Design review of the part built by this model. Coordinates are the model's own, in mm. A direction names the side the tool comes from. Give positions to 0.01 mm unless a question says otherwise; leave off trailing zeros. Loops run counter-clockwise (first coordinate to the right, second up) from the corner with the lowest first, then second, coordinate; pieces in that order, holes last. Notation, with made-up numbers: (58.25, 10.25) -> (82.25, 10.25) arc R9 cw to (82.25, 20.25) -> close; hole circle Ø9 at (13, -35.5). An arc over 180 degrees is marked (long way). Answer in a Markdown table with one row per item. Add a question column.
(1) For faces 1 (the flat face through (-15.24, 12, -2)), 2 (the flat face through (-16, -7, -3.175)), list the 3-axis set-ups (+Z, -Z, +X, -X, +Y, -Y) from which the entire face can be reached by the end or side of a thin tool; tool diameter is ignored.
(2) For line 1 (Y direction, x = -25.4, z = -0.95); line 2 (Y direction, x = 0, z = -2.4); line 3 (X direction, y = 6.5, z = -2) (3 decimals), list the stretches that pass through material, from the lowest coordinate up.
(3) Consider section D-D on y = 6.35. Write out the cut boundary in (x, z) (3 decimals), then the cut area to 3 significant figures.
(4) Consider section C-C on x = 12.7. Write out the cut boundary in (y, z) (3 decimals), then the cut area to 3 significant figures.
(5) Draft analysis for pull direction Y (two halves, no side actions). For faces 3 (the cylindrical face through (-23.026, 7.098, -1.565)), 4 (the flat face through (-8, -14, 0)), 5 (the cylindrical face through (-23.026, -5.602, -1.565)), 6 (the cylindrical face through (33.493, -30.392, -1.61)), state which applies: +Y half, -Y half, draft (parallel to the pull), parting line (faces both ways), or undercut.
(6) Consider section B-B on y = -19.05. Write out the cut boundary in (x, z) (1 decimal), then the cut area to 3 significant figures.
(7) For pin 1 (4.5 mm diameter, centred on x = 25.4, y = -19.05, fed in from +Z), flat-tipped, find the tip position at first contact; note if it passes through.
(8) Consider section A-A on x = -25.4. Write out the cut boundary in (y, z) (3 decimals).
from build123d import *

# Parameters (mm, degrees)
SKETCH1_R                                       = 2.4892
BASE_FLANGE1_DEPTH                              = 3.175
FILLET2_R                                       = 4.7625
CSK_FOR_10_FLAT_HEAD_MACHINE_SCREW1_D           = 5.1054
CSK_FOR_10_FLAT_HEAD_MACHINE_SCREW1_DEPTH       = 19.05
CSK_FOR_10_FLAT_HEAD_MACHINE_SCREW1_CSINK_D     = 9.779
CSK_FOR_10_FLAT_HEAD_MACHINE_SCREW1_CSINK_ANGLE = 82
CSK_FOR_10_FLAT_HEAD_MACHINE_SCREW1_TIP         = 1.533816902


# Sheet-metal steps are written as plain solids
with BuildPart() as part:
    # Sketch1 → Base-Flange1 (new body)
    with BuildSketch(Plane.XY):
        Polygon((-15.24, 31.75), (-34.925, 31.75), (-34.925, -31.75), (34.925, -31.75), (34.925, -7.62), (-15.24, -7.62), align=None)
        with Locations((-25.4, -6.35)):
            Circle(SKETCH1_R, mode=Mode.SUBTRACT)
        with Locations((-25.4, 6.35)):
            Circle(SKETCH1_R, mode=Mode.SUBTRACT)
        with Locations((0, -19.05)):
            Circle(SKETCH1_R, mode=Mode.SUBTRACT)
        with Locations((12.7, -19.05)):
            Circle(SKETCH1_R, mode=Mode.SUBTRACT)
        with Locations((25.4, -19.05)):
            Circle(SKETCH1_R, mode=Mode.SUBTRACT)
    extrude(amount=-BASE_FLANGE1_DEPTH)

    # Fillet2
    fillet2_edges = [part.edges().sort_by_distance(p)[0] for p in [
        (-34.925, -31.75, -1.5875),
        (34.925, -31.75, -1.5875),
        (34.925, -7.62, -1.5875),
        (-15.24, -7.62, -1.5875),
        (-15.24, 31.75, -1.5875),
        (-34.925, 31.75, -1.5875),
    ]]
    fillet(fillet2_edges, radius=FILLET2_R)

    # CSK for #10 Flat Head Machine Screw1
    with Locations(Plane(origin=(0, 0, -3.175), x_dir=(-1, 0, 0), z_dir=(0, 0, -1))):
        with Locations((-25.4, -19.05)):
            CounterSinkHole(CSK_FOR_10_FLAT_HEAD_MACHINE_SCREW1_D / 2, CSK_FOR_10_FLAT_HEAD_MACHINE_SCREW1_CSINK_D / 2, depth=CSK_FOR_10_FLAT_HEAD_MACHINE_SCREW1_DEPTH, counter_sink_angle=CSK_FOR_10_FLAT_HEAD_MACHINE_SCREW1_CSINK_ANGLE)
            with Locations((0, 0, -(CSK_FOR_10_FLAT_HEAD_MACHINE_SCREW1_DEPTH + CSK_FOR_10_FLAT_HEAD_MACHINE_SCREW1_TIP / 2))):  # 118° drill point
                Cone(0, CSK_FOR_10_FLAT_HEAD_MACHINE_SCREW1_D / 2, CSK_FOR_10_FLAT_HEAD_MACHINE_SCREW1_TIP, mode=Mode.SUBTRACT)


solid = part.part
Values follow:
| question | item | result |
|---|---|---|
| 1 | face 1 | +Z, -Z, +X, +Y |
| 1 | face 2 | -Z, +X, -X, +Y, -Y |
| 2 | line 1 | -31.75 to -8.84, -3.86 to 3.86, 8.84 to 31.75 |
| 2 | line 2 | -31.75 to -21.54, -16.56 to -7.62 |
| 2 | line 3 | -34.925 to -27.885, -22.915 to -15.24 |
| 3 | outline | (-34.925, -3.175) -> (-27.889, -3.175) -> (-27.889, 0) -> (-34.925, 0) -> close; (-22.911, -3.175) -> (-15.24, -3.175) -> (-15.24, 0) -> (-22.911, 0) -> close |
| 3 | area | 46.7 mm2 |
| 4 | outline | (-31.75, -3.175) -> (-21.539, -3.175) -> (-21.539, 0) -> (-31.75, 0) -> close; (-16.561, -3.175) -> (-7.62, -3.175) -> (-7.62, 0) -> (-16.561, 0) -> close |
| 4 | area | 60.8 mm2 |
| 5 | face 3 | undercut |
| 5 | face 4 | draft |
| 5 | face 5 | undercut |
| 5 | face 6 | -Y half |
| 6 | outline | (-34.9, -3.2) -> (-2.5, -3.2) -> (-2.5, 0) -> (-34.9, 0) -> close; (2.5, -3.2) -> (10.2, -3.2) -> (10.2, 0) -> (2.5, 0) -> close; (15.2, -3.2) -> (20.5, -3.2) -> (22.8, -0.5) -> (22.8, 0) -> (15.2, 0) -> close; (28, -0.5) -> (30.3, -3.2) -> (34.9, -3.2) -> (34.9, 0) -> (28, 0) -> close |
| 6 | area | 168 mm2 |
| 7 | pin 1 | through |
| 8 | outline | (-31.75, -3.175) -> (-8.839, -3.175) -> (-8.839, 0) -> (-31.75, 0) -> close; (-3.861, -3.175) -> (3.861, -3.175) -> (3.861, 0) -> (-3.861, 0) -> close; (8.839, -3.175) -> (31.75, -3.175) -> (31.75, 0) -> (8.839, 0) -> close |
